Verification items for the finished model (mm, model axes). Face numbers are marked on the shaded views. A direction names the side the tool comes from. Give positions to 0.01 mm unless a question says otherwise; leave off trailing zeros. Write each loop counter-clockwise with the first axis right and the second up, starting at its lowest first coordinate (ties: lowest second). Pieces come first, ordered by that corner, then holes. Notation, with made-up numbers: (-13, 41.25) -> (31, 41.25) arc R20 ccw to (31, 59.25) -> close; hole circle Ø5 at (73.5, 44). An arc over 180 degrees is marked (long way). Use one line per item in the form item = value. Start each with the question number.
(1) Release check for a two-part mould opening along Y. For the marked faces 1, 2 and 3 record: pulls with the +Y half, pulls with the -Y half, needs draft (parallel to the pull), parting line crosses it, or undercut.
(2) Scan lines: L1, parallel to Y at x = 1.4, z = 0; L2, parallel to Z at x = 2.6, y = 0.5; L3, parallel to X at y = -11, z = 4.5. Record each from-to range of solid material in increasing order.
(3) Depth check by flat-ended pin: pin 1 Ø3 at (y, z) = (0, 5) entering from -X; pin 2 Ø5 at (y, z) = (-12, 0) entering from -X. Enter the tip coordinate at first touch or a pass-through.
(4) Section check A-A, the plane y = 0. Record the cut outline in (x, z).
(5) Section check C-C, the plane x = 2.3. State how many separate pieces and enclosed holes the cut face has, plus the area to 3 significant figures.
(6) Section check D-D, the plane z = 12. Record the cut outline in (x, y), plus the area to 3 significant figures.
(7) Set-up check for the marked faces 4 and 5: record each of +Z, -Z, +X, -X, +Y, -Y from which the full face is reachable in a straight line by a thin tool's end or side.
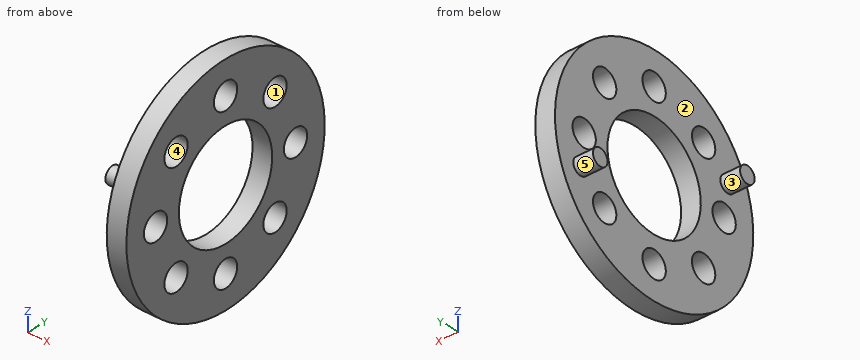
from build123d import *

# Parameters (mm, degrees)
SKETCH1_R           = 17
SKETCH1_R_2         = 2
SKETCH1_R_3         = 8
BOSS_EXTRUDE1_DEPTH = 3
SKETCH2_R           = 1.25
BOSS_EXTRUDE2_DEPTH = 3


with BuildPart() as part:
    # Sketch1 → Boss-Extrude1 (new body)
    with BuildSketch(Plane(origin=(0, 0, 0), x_dir=(0, 0, -1), z_dir=(1, 0, 0))):
        Circle(SKETCH1_R)
        with Locations((0, 12)):
            Circle(SKETCH1_R_2, mode=Mode.SUBTRACT)
        with Locations((8.485281374, 8.485281374)):
            Circle(SKETCH1_R_2, mode=Mode.SUBTRACT)
        with Locations((12, 0)):
            Circle(SKETCH1_R_2, mode=Mode.SUBTRACT)
        with Locations((8.485281374, -8.485281374)):
            Circle(SKETCH1_R_2, mode=Mode.SUBTRACT)
        with Locations((0, -12)):
            Circle(SKETCH1_R_2, mode=Mode.SUBTRACT)
        with Locations((-8.485281374, -8.485281374)):
            Circle(SKETCH1_R_2, mode=Mode.SUBTRACT)
        with Locations((-12, 0)):
            Circle(SKETCH1_R_2, mode=Mode.SUBTRACT)
        with Locations((-8.485281374, 8.485281374)):
            Circle(SKETCH1_R_2, mode=Mode.SUBTRACT)
        Circle(SKETCH1_R_3, mode=Mode.SUBTRACT)
    extrude(amount=BOSS_EXTRUDE1_DEPTH)

    # Sketch2 → Boss-Extrude2 (add)
    with BuildSketch(Plane.ZY):
        with Locations(Location((-4.818635741, 12.610739455, 0), (0, 0, 180))):
            Circle(SKETCH2_R)
        with Locations(Location((4.818635741, -12.610739455, 0), (0, 0, 180))):
            Circle(SKETCH2_R)
    extrude(amount=BOSS_EXTRUDE2_DEPTH)


solid = part.part
Completed:
q1.face_1 = undercut
q1.face_2 = needs draft
q1.face_3 = parting line crosses it
q2.L1 = -17 to -14, -10 to -8, 8 to 10, 14 to 17
q2.L2 = -16.99 to -13.94, -10.06 to -7.98, 7.98 to 10.06, 13.94 to 16.99
q2.L3 = 0 to 3
q3.pin_1 = through
q3.pin_2 = 0
q4.outline = (0, -17) -> (3, -17) -> (3, -14) -> (0, -14) -> close; (0, -10) -> (3, -10) -> (3, -8) -> (0, -8) -> close; (0, 8) -> (3, 8) -> (3, 10) -> (0, 10) -> close; (0, 14) -> (3, 14) -> (3, 17) -> (0, 17) -> close
q5.separate_pieces = 1
q5.enclosed_holes = 9
q5.area = 606 mm²
q6.outline = (0, -12.04) -> (3, -12.04) -> (3, -2) -> (0, -2) -> close; (0, 2) -> (3, 2) -> (3, 12.04) -> (0, 12.04) -> close
q6.area = 60.2 mm²
q7.face_4 = +X, -X
q7.face_5 = -X
